```python
from build123d import *

# Parameters (mm, degrees)
F1_R     = 14.2875
F2_DEPTH = 25.4
F0_R     = 14.2875
F0_R_2   = 10.9982
F3_DEPTH = 19.05


with BuildPart() as f2:
    # F1 (on Front) → F2 (new body)
    with BuildSketch(Plane.XZ):
        with BuildLine():
            ThreePointArc((13.8718760728, 28.3289313848), (0, 17.4625), (-13.8718760728, 28.3289313848))
            ThreePointArc((-13.8718760728, 28.3289313848), (-16.5359438351, 9.5470316245), (-31.4695122777, -2.1510686152))
            ThreePointArc((-31.4695122777, -2.1510686152), (-18.912441482, -4.4535326513), (-13.2088065702, -15.875))
            ThreePointArc((-13.2088065702, -15.875), (-14.3517276668, -21.4743483284), (-17.5976362049, -26.1778627696))
            ThreePointArc((-17.5976362049, -26.1778627696), (0, -19.094063249), (17.5976362049, -26.1778627696))
            ThreePointArc((17.5976362049, -26.1778627696), (15.1229686136, -8.73125), (31.4695122777, -2.1510686152))
            ThreePointArc((31.4695122777, -2.1510686152), (16.5359438351, 9.5470316245), (13.8718760728, 28.3289313848))
        make_face()
        Circle(F1_R, mode=Mode.SUBTRACT)
    extrude(amount=F2_DEPTH)

    # F0 (on Front) → F3 (join)
    with BuildSketch(Plane.XZ):
        with Locations((0, 31.75)):
            Circle(F0_R)
        with Locations((0, 31.75)):
            Circle(F0_R_2, mode=Mode.SUBTRACT)
        with Locations((27.4963065702, -15.875)):
            Circle(F0_R)
        with Locations((27.4963065702, -15.875)):
            Circle(F0_R_2, mode=Mode.SUBTRACT)
        with Locations((-27.4963065702, -15.875)):
            Circle(F0_R)
        with Locations((-27.4963065702, -15.875)):
            Circle(F0_R_2, mode=Mode.SUBTRACT)
    extrude(amount=F3_DEPTH)


solid = f2.part
```
Check sheet for the modelled part. Datum: model origin and axes. Units: mm. A direction names the side the tool comes from. Give positions to 0.01 mm unless a question says otherwise; leave off trailing zeros. Order: outer loops, then holes, each group sorted by start corner. A loop starts at its lowest first (then second) coordinate and runs counter-clockwise, first axis right, second up. Notation, with made-up numbers: M 72.5,-22.5 L 129.5,-22.5 A5 ccw 129.5,-16.5 Z; hole C 61,59 d8. An arc over 180 degrees is marked long. Answer in a Markdown table with one row per item. Add a question column.
Q1. Sectioned sample at C-C, the plane x = 0. Record the boundary of the cut face in (y, z), and give its area (3 significant figures).
Q2. Sectioned sample at A-A, the plane y = -12. Count the separate pieces of the cut face and the enclosed holes in it, and give its area (3 significant figures).
Q3. Thickness scan on L1, parallel to X at y = -6.5, z = -16; L2, parallel to Z at x = 8.5, y = -10.25; L3, parallel to X at y = -7.25, z = -9. Record the ranges inside material, lowest first.
Q4. Gauge pin test, flat ends, axial feed: pin 1 Ø8 at (y, z) = (-14.5, 28.5) entering from +X; pin 2 Ø2 at (x, y) = (-1, -8) entering from -Z; pin 3 Ø4 at (y, z) = (-16.5, 9.5) entering from -X. Record the tip position at first contact, or that the pin passes through.
Q5. Sectioned sample at B-B, the plane z = 22. Record the boundary of the cut face in (x, y).
Q6. Access from +Z, -Z, +X, -X, +Y, -Y to the whole of each face (thin tool, end or side, straight path). Record for faces 5 (the flat face through (7, -19.05, 23)), 6 (the cylindrical face through (14.992, -22.181, -8.963)), 7 (the cylindrical face through (-14.274, -12.522, 0.628)).
Q7. Release check for a two-part mould opening along X. For faces 1 (the flat face through (-9.5, 0, 10.9)), 2 (the cylindrical face through (-16.401, -12.522, 9.783)), 3 (the cylindrical face through (0.363, -9.392, 46.033)), 4 (the cylindrical face through (18.77, -9.39, -22.57)) record: released by +X, released by -X, zero draft, split by the parting line, or undercut.
Verdict:
| question | item | result |
|---|---|---|
| 1 | outline | M -25.4,-19.09 L 0,-19.09 L 0,-14.29 L -25.4,-14.29 Z; M -25.4,14.29 L 0,14.29 L 0,20.75 L -19.05,20.75 L -19.05,17.46 L -25.4,17.46 Z; M -19.05,42.75 L 0,42.75 L 0,46.04 L -19.05,46.04 Z |
| 1 | area | 328 mm² |
| 2 | separate pieces | 1 |
| 2 | enclosed holes | 4 |
| 2 | area | 1,520 mm² |
| 3 | L1 | -41.78 to -38.49, -16.5 to 16.5, 38.49 to 41.78 |
| 3 | L2 | -20.56 to -11.48, 11.48 to 24.77, 38.73 to 43.23 |
| 3 | L3 | -40.02 to -36.08, -18.91 to -11.1, 11.1 to 18.91, 36.08 to 40.02 |
| 4 | pin 1 | x = 14.29 |
| 4 | pin 2 | z = -19.17 |
| 4 | pin 3 | x = -17.85 |
| 5 | outline | M -13.13,-25.4 L -10.44,-25.4 L -10.44,-19.05 L -5.09,-19.05 L -5.09,0 L -13.13,0 Z; M 5.09,-19.05 L 10.44,-19.05 L 10.44,-25.4 L 13.13,-25.4 L 13.13,0 L 5.09,0 Z |
| 6 | face 5 | +Z, -Y |
| 6 | face 6 | -Y |
| 6 | face 7 | +Y, -Y |
| 7 | face 1 | zero draft |
| 7 | face 2 | released by -X |
| 7 | face 3 | split by the parting line |
| 7 | face 4 | undercut |
